Source: three-view drawing plus pictorial views. Frame: mm from the lowest corner of the part. Round coordinates to 2 decimals unless told otherwise and drop trailing zeros. Write each loop counter-clockwise with the first axis right and the second up, starting at its lowest first coordinate (ties: lowest second). Pieces come first, ordered by that corner, then holes. Notation, with made-up numbers: M -13,-19 L -6,-19 A20 ccw -6,11 Z; hole C -36,52 d3. An arc over 180 degrees is marked long. Answer as CSV lines item,"result". Start each with the question number.
Q1. Section query D-D on x = 7. Output: boundary loops of the cut face in (y, z).
Q2. First-contact query: pin 1 (2 mm diameter, centred on x = 7, z = 7, fed in from +Y). Flat tip, straight axial feed; report the tip coordinate or a pass-through.
Q3. Section query C-C on y = 1.9. Output: boundary loops of the cut face in (x, z).
Q4. Ray query, probe 1 along X at (y, z) = (2.1, 7); probe 2 along X at (y, z) = (2.65, 6); probe 3 along X at (y, z) = (2.75, 25.5). Return the intervals inside material, ascending.
Q5. Section query A-A on z = 25. Output: boundary loops of the cut face in (x, y).
Q6. Section query B-B on x = 25. Output: boundary loops of the cut face in (y, z), and give its area (3 significant figures).
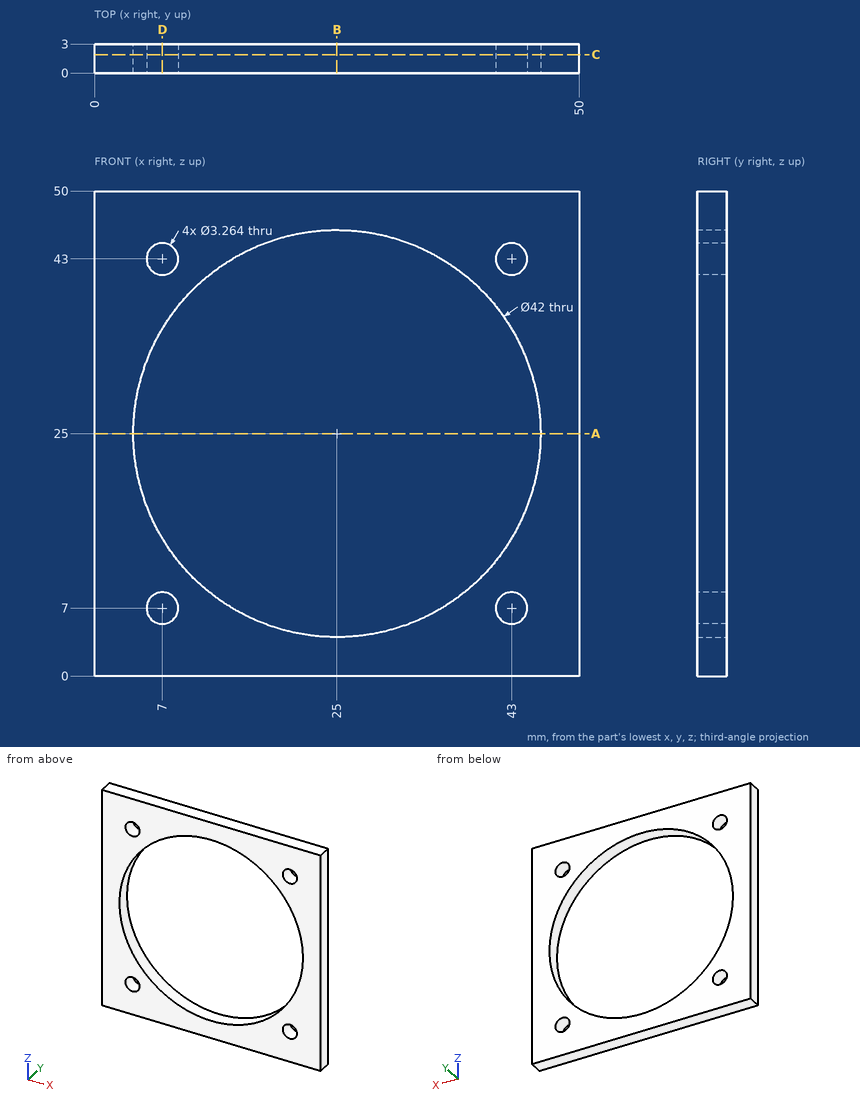
Entries:
1,outline,"M 0,0 L 3,0 L 3,5.37 L 0,5.37 Z; M 0,8.63 L 3,8.63 L 3,14.18 L 0,14.18 Z; M 0,35.82 L 3,35.82 L 3,41.37 L 0,41.37 Z; M 0,44.63 L 3,44.63 L 3,50 L 0,50 Z"
2,pin 1,"passes through"
3,outline,"M 0,0 L 50,0 L 50,50 L 0,50 Z; hole C 25,25 d42; hole C 7,7 d3.26; hole C 7,43 d3.26; hole C 43,7 d3.26; hole C 43,43 d3.26"
4,probe 1,"x = 0 to 5.37, 8.63 to 14.18, 35.82 to 41.37, 44.63 to 50"
4,probe 2,"x = 0 to 5.71, 8.29 to 16.06, 33.94 to 41.71, 44.29 to 50"
4,probe 3,"x = 0 to 4.01, 45.99 to 50"
5,outline,"M 0,0 L 4,0 L 4,3 L 0,3 Z; M 46,0 L 50,0 L 50,3 L 46,3 Z"
6,outline,"M 0,0 L 3,0 L 3,4 L 0,4 Z; M 0,46 L 3,46 L 3,50 L 0,50 Z"
6,area,"24.0 mm^2"
